from build123d import *

# Parameters (mm, degrees)
EXTRUDE_2_DEPTH     = 5
SKETCH_3_R          = 1.65
CUT_EXTRUDE_1_DEPTH = 10


with BuildPart() as part:
    # Эскиз1 → Бобышка-Вытянуть2 (new body)
    with BuildSketch(Plane(origin=(139.725199601, 79.945164962, 32.467820781), x_dir=(-1, 0, 0), z_dir=(0, 0, -1))):
        Polygon((-54.33719348, 85.310831528), (-54.33719348, 195.310831528), (-19.33719348, 195.310831528), (-19.33719348, 205.310831528), (-34.368760963, 223.252548998), (-254.305625996, 223.252548998), (-269.33719348, 205.310831528), (-269.33719348, 195.310831528), (-234.33719348, 195.310831528), (-234.33719348, 85.310831528), (-269.33719348, 85.310831528), (-269.33719348, 75.310831528), (-184.33719348, 60.310831528), (-104.33719348, 60.310831528), (-19.33719348, 75.310831528), (-19.33719348, 85.310831528), align=None)
    extrude(amount=EXTRUDE_2_DEPTH)

    # Эскиз3 → Вырез-Вытянуть1 (cut)
    with BuildSketch(Plane(origin=(0, 0, 27.467820781), x_dir=(-1, 0, 0), z_dir=(0, 0, -1))):
        with Locations((-217.562393081, 177.75599649)):
            Circle(SKETCH_3_R)
        with Locations((-350.562393081, 177.75599649)):
            Circle(SKETCH_3_R)
        with Locations((-356.614117219, 264.25599649)):
            Circle(SKETCH_3_R)
        with Locations((-344.510668943, 251.25599649)):
            Circle(SKETCH_3_R)
        with Locations((-211.510668943, 251.25599649)):
            Circle(SKETCH_3_R)
        with Locations((-223.614117219, 264.25599649)):
            Circle(SKETCH_3_R)
    extrude(amount=-CUT_EXTRUDE_1_DEPTH, mode=Mode.SUBTRACT)


solid = part.part
Verification items for the finished model (mm, model axes). A direction names the side the tool comes from. Round coordinates to 2 decimals unless told otherwise and drop trailing zeros. Order: outer loops, then holes, each group sorted by start corner. A loop starts at its lowest first (then second) coordinate and runs counter-clockwise, first axis right, second up. Notation, with made-up numbers: (51.25, 39) -> (107.25, 39) arc R19 ccw to (107.25, 63) -> close; hole circle Ø6 at (73.5, -39.5). An arc over 180 degrees is marked (long way). Put each result on its own line as item: value.
1) Section check D-D (x = 206.5). Record the cut outline in (y, z), then the cut area to 3 significant figures.
Final values:
outline: (146.88, 27.47) -> (303.2, 27.47) -> (303.2, 32.47) -> (146.88, 32.47) -> close
area: 782 mm^2
2) Section check C-C (y = 231.5). Record the cut outline in (x, z).
Final values:
outline: (194.06, 27.47) -> (374.06, 27.47) -> (374.06, 32.47) -> (194.06, 32.47) -> close
3) Section check A-A (x = 379). Record the cut outline in (y, z), then the cut area to 3 significant figures.
Final values:
outline: (149.95, 27.47) -> (165.26, 27.47) -> (165.26, 32.47) -> (149.95, 32.47) -> close; (275.26, 27.47) -> (303.2, 27.47) -> (303.2, 32.47) -> (275.26, 32.47) -> close
area: 216 mm^2
4) Material ranges on line 1 (X direction, y = 174, z = 29.05); line 2 (Y direction, x = 377.5, z = 31.55); line 3 (Y direction, x = 193, z = 30), recorded low to high.
Final values:
line 1: x = 194.06 to 374.06
line 2: y = 149.69 to 165.26, 275.26 to 303.2
line 3: y = 149.27 to 165.26, 275.26 to 303.2
5) Set-up check for faces 1 (the flat face through (286, 223, 32.468)), 2 (the flat face through (176, 165.256, 30)), 3 (the flat face through (392, 275.256, 30)): record each of +Z, -Z, +X, -X, +Y, -Y from which the full face is reachable in a straight line by a thin tool's end or side.
Final values:
face 1: +Z, +X, -X, +Y, -Y
face 2: +Z, -Z, -X
face 3: +Z, -Z, +X
6) Depth check by flat-ended pin: pin 1 (1 mm diameter, centred on x = 184.5, z = 30.5, fed in from -Y); pin 2 (2 mm diameter, centred on x = 217.56, y = 177.76, fed in from +Z); pin 3 (2.5 mm diameter, centred on x = 177, z = 30.5, fed in from -Y); pin 4 (2.5 mm diameter, centred on x = 394, z = 29, fed in from -Y). Enter the tip coordinate at first touch or a pass-through.
Final values:
pin 1: stops at y = 150.68
pin 2: passes through
pin 3: stops at y = 151.87
pin 4: stops at y = 152.38
7) Section check B-B (z = 28.35). Record the cut outline in (x, y).
Final values:
outline: (159.06, 155.26) -> (244.06, 140.26) -> (324.06, 140.26) -> (409.06, 155.26) -> (409.06, 165.26) -> (374.06, 165.26) -> (374.06, 275.26) -> (409.06, 275.26) -> (409.06, 285.26) -> (394.03, 303.2) -> (174.09, 303.2) -> (159.06, 285.26) -> (159.06, 275.26) -> (194.06, 275.26) -> (194.06, 165.26) -> (159.06, 165.26) -> close; hole circle Ø3.3 at (211.51, 251.26); hole circle Ø3.3 at (217.56, 177.76); hole circle Ø3.3 at (223.61, 264.26); hole circle Ø3.3 at (344.51, 251.26); hole circle Ø3.3 at (350.56, 177.76); hole circle Ø3.3 at (356.61, 264.26)
